Can you work these out from the drawing? Everything is in mm from the part's minimum corner. A direction names the side the tool comes from. Coordinates: 2 decimals unless noted, no trailing zeros. Order: outer loops, then holes, each group sorted by start corner. A loop starts at its lowest first (then second) coordinate and runs counter-clockwise, first axis right, second up. Notation, with made-up numbers: (-40, 61) - (-21, 61) arc R23 ccw to (-21, 75) - close; hole circle Ø4 at (3.5, 49). An arc over 180 degrees is marked (long way). Answer as CSV lines item,"result". Start each with the question number.
Q1. For pin 1 Ø2.5 at (y, z) = (4, 13.5) entering from +X; pin 2 Ø20 at (x, z) = (50, 33) entering from +Y, each with a flat end and sliding along its axis, tell me the tip position at first contact or that it passes through.
Q2. Suppose I cut it at C-C (y = 7). Please give me the cut outline in (x, z), then the cut area to 3 significant figures.
Q3. Suppose I cut it at B-B (z = 41). Please give me the cut outline in (x, y).
Q4. For the marked faces 1 and 2, which set-ups out of +Z, -Z, +X, -X, +Y, -Y let a thin tool reach every point of the face, with its end or its side?
Q5. I need wall thicknesses on line 1 (Y direction, x = 24.5, z = 29); line 2 (Z direction, x = 43, y = 1.5); line 3 (Z direction, x = 9.5, y = 5.5). Which ranges of each line are inside material? Lowest first, please.
Q6. Suppose I cut it at D-D (y = 3). Please give me the cut outline in (x, z).
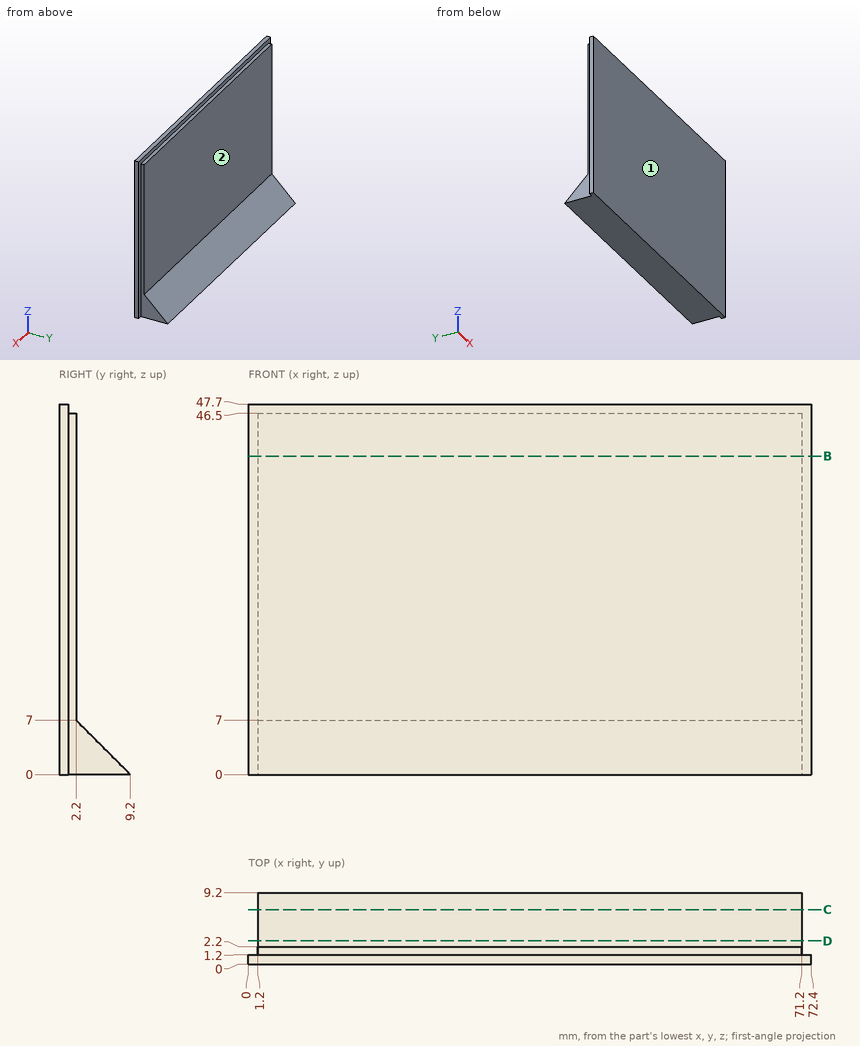
Here are the results:
1,pin 1,"passes through"
1,pin 2,"stops at y = 2.2"
2,outline,"(1.2, 0) - (71.2, 0) - (71.2, 2.2) - (1.2, 2.2) - close"
2,area,"154 mm²"
3,outline,"(0, 0) - (72.4, 0) - (72.4, 1.2) - (71.2, 1.2) - (71.2, 2.2) - (1.2, 2.2) - (1.2, 1.2) - (0, 1.2) - close"
4,face 1,"+Z, -Z, +X, -X, -Y"
4,face 2,"+Z, +X, -X, +Y"
5,line 1,"y = 0 to 2.2"
5,line 2,"z = 0 to 46.5"
5,line 3,"z = 0 to 3.7"
6,outline,"(1.2, 0) - (71.2, 0) - (71.2, 6.2) - (1.2, 6.2) - close"
